```python
from build123d import *

# Parameters (mm, degrees)
F0_W     = 60
F0_H     = 60
F1_DEPTH = 12
F3_DEPTH = 12
F4_W     = 50
F4_H     = 23
F5_DEPTH = 20
F7_DEPTH = 20
F8_R     = 12.5
F9_DEPTH = 20


with BuildPart() as f1:
    # F0 (on Front) → F1 (new body)
    with BuildSketch(Plane.XZ):
        Rectangle(F0_W, F0_H)
    extrude(amount=F1_DEPTH)

    # F2 (on face) → F3 (join)
    with BuildSketch(Plane.XY.offset(30)):
        Polygon((-30, 103), (-30, 0), (30, 0), (-10, 103), align=None)
    extrude(amount=-F3_DEPTH)

    # F4 (on face) → F5 (join)
    with BuildSketch(Plane(origin=(-30, 0, 0), x_dir=(0, -1, 0), z_dir=(-1, 0, 0))):
        with Locations((-78, 6.5)):
            Rectangle(F4_W, F4_H)
    extrude(amount=-F5_DEPTH)

    # F6 (on face) → F7 (join)
    with BuildSketch(Plane(origin=(-30, 0, 0), x_dir=(0, -1, 0), z_dir=(-1, 0, 0))):
        with BuildLine():
            Line((-53, -5), (-103, -5))
            ThreePointArc((-103, -5), (-78, -30), (-53, -5))
        make_face()
    extrude(amount=-F7_DEPTH)

    # F8 (on face) → F9 (cut)
    with BuildSketch(Plane(origin=(-30, 0, 0), x_dir=(0, -1, 0), z_dir=(-1, 0, 0))):
        with Locations((-78, -5)):
            Circle(F8_R)
    extrude(amount=-F9_DEPTH, mode=Mode.SUBTRACT)


solid = f1.part
```
Input: part model. Units: mm. Frame: model coordinates. A direction names the side the tool comes from. Coordinates: 2 decimals unless noted, no trailing zeros. Loops run counter-clockwise (first coordinate to the right, second up) from the corner with the lowest first, then second, coordinate; pieces in that order, holes last. Notation, with made-up numbers: (71, -12) -> (114, -12) arc R34 cw to (114, 24) -> close; hole circle Ø1 at (11, -39.75). An arc over 180 degrees is marked (long way). Use a Markdown table: item, result.
1) Cut plane B-B (x = -20.5). Return the cut outline in (y, z).
Results found:
| item | result |
|---|---|
| outline | (-12, -30) -> (0, -30) -> (0, 18) -> (53, 18) -> (53, -5) arc R25 ccw to (103, -5) -> (103, 30) -> (-12, 30) -> close; hole circle Ø25 at (78, -5) |
2) Cut plane C-C (z = -8). Return the cut outline in (x, y).
Results found:
| item | result |
|---|---|
| outline | (-30, -12) -> (30, -12) -> (30, 0) -> (-30, 0) -> close; (-30, 53.18) -> (-10, 53.18) -> (-10, 65.87) -> (-30, 65.87) -> close; (-30, 90.13) -> (-10, 90.13) -> (-10, 102.82) -> (-30, 102.82) -> close |
3) Material intervals for line 1 along Y through (x, z) = (-23, 14); line 2 along Y through (x, z) = (-13, -16); line 3 along Z through (x, y) = (-20.5, 78), sorted ascending. Write a range as from..to.
Results found:
| item | result |
|---|---|
| line 1 | y = -12..0, 53..103 |
| line 2 | y = -12..0, 55.55..72.06, 83.94..100.45 |
| line 3 | z = -30..-17.5, 7.5..30 |
4) Contact query for flat-ended pins moving along their axis: pin 1 (6 mm diameter, centred on x = 19, y = 22.5, fed in from -Z); pin 2 (8 mm diameter, centred on y = 77, z = -11.5, fed in from -X); pin 3 (2 mm diameter, centred on x = 18, z = 3.5, fed in from +Y). Output: stop coordinate, or through.
Results found:
| item | result |
|---|---|
| pin 1 | stops at z = 18 |
| pin 2 | passes through |
| pin 3 | stops at y = 0 |
5) Access query for faces 4 (the flat face through (-10, 89.5, -11)), 5 (the flat face through (0, -6, -30)), 6 (the flat face through (0, 0, -6)). Directions: +Z, -Z, +X, -X, +Y, -Y. A direction counts if a zero-diameter tool reaches every point of the face in a straight line with its end or side. Return the directions, or none.
Results found:
| item | result |
|---|---|
| face 4 | -Z, +X, +Y |
| face 5 | -Z, +X, -X, +Y, -Y |
| face 6 | -Z, +X, -X |
6) Pull-direction query (Y, two-part tool) for faces 1 (the flat face through (-7, 34, 30)), 2 (the flat face through (0, -12, 0)), 3 (the cylindrical face through (-20.14, 78.55, -29.994)); classes: released by +Y, released by -Y, zero draft, split by the parting line, or undercut.
Results found:
| item | result |
|---|---|
| face 1 | zero draft |
| face 2 | released by -Y |
| face 3 | undercut |
7) Cut plane D-D (x = 10). Return the cut outline in (y, z).
Results found:
| item | result |
|---|---|
| outline | (-12, -30) -> (0, -30) -> (0, 18) -> (51.5, 18) -> (51.5, 30) -> (-12, 30) -> close |
8) Cut plane A-A (y = 78). Return the cut outline in (x, z), then the cut area to 3 significant figures.
Results found:
| item | result |
|---|---|
| outline | (-30, -30) -> (-10, -30) -> (-10, -17.5) -> (-30, -17.5) -> close; (-30, 7.5) -> (-10, 7.5) -> (-10, 18) -> (-0.29, 18) -> (-0.29, 30) -> (-30, 30) -> close |
| area | 817 mm2 |
